from build123d import *

# Parameters (mm, degrees)
SKETCH_1_W          = 100
SKETCH_1_H          = 65
EXTRUDE_1_DEPTH     = 12
SKETCH_2_R          = 3.5
CUT_EXTRUDE_2_DEPTH = 10
SKETCH_3_R          = 3.5
CUT_EXTRUDE_3_DEPTH = 61.466933112
SKETCH_4_R          = 3.5
CUT_EXTRUDE_4_DEPTH = 61.466933112
CUT_EXTRUDE_5_REACH = 84.879
SKETCH_5_R          = 1.5
CUT_EXTRUDE_6_REACH = 84.879
SKETCH_6_R          = 1.5
FILLET_3_R          = 2


with BuildPart() as part:
    # 草图1 → 凸台-拉伸1 (new body)
    with BuildSketch(Plane(origin=(0, 0, 0), x_dir=(1, 0, 0), z_dir=(0, 1, 0))):
        Rectangle(SKETCH_1_W, SKETCH_1_H)
    extrude(amount=EXTRUDE_1_DEPTH)

    # 草图2 → 切除-拉伸2 (cut)
    with BuildSketch(Plane(origin=(0, 12, 0), x_dir=(1, 0, 0), z_dir=(0, 1, 0))):
        with Locations(Location((-40, -9, 0), (0, 0, 270))):
            Circle(SKETCH_2_R)
        with Locations(Location((40, -9, 0), (0, 0, 90))):
            Circle(SKETCH_2_R)
        with BuildLine():
            Line((-30.422291236, 30.788854382), (-33.577708764, 29.211145618))
            ThreePointArc((-33.577708764, 29.211145618), (-34.012630114, 29.053502021), (-34.472135955, 29))
            Line((-34.472135955, 29), (-41, 29))
            ThreePointArc((-41, 29), (-43.828427125, 27.828427125), (-45, 25))
            Line((-45, 25), (-45, 6))
            ThreePointArc((-45, 6), (-43.535533906, 2.464466094), (-40, 1))
            ThreePointArc((-40, 1), (-30, -9), (-40, -19))
            ThreePointArc((-40, -19), (-45, -24), (-40, -29))
            Line((-40, -29), (-34.439229319, -29))
            ThreePointArc((-34.439229319, -29), (-33.976113717, -29.054357705), (-33.538172016, -29.214476061))
            Line((-33.538172016, -29.214476061), (-30.425003094, -30.785523939))
            ThreePointArc((-30.425003094, -30.785523939), (-29.987061393, -30.945642295), (-29.52394579, -31))
            Line((-29.52394579, -31), (29.52394579, -31))
            ThreePointArc((29.52394579, -31), (29.987061393, -30.945642295), (30.425003094, -30.785523939))
            Line((30.425003094, -30.785523939), (33.538172016, -29.214476061))
            ThreePointArc((33.538172016, -29.214476061), (33.976113717, -29.054357705), (34.439229319, -29))
            Line((34.439229319, -29), (40, -29))
            ThreePointArc((40, -29), (45, -24), (40, -19))
            ThreePointArc((40, -19), (30, -9), (40, 1))
            ThreePointArc((40, 1), (43.535533906, 2.464466094), (45, 6))
            Line((45, 6), (45, 25))
            ThreePointArc((45, 25), (43.828427125, 27.828427125), (41, 29))
            Line((41, 29), (34.472135955, 29))
            ThreePointArc((34.472135955, 29), (34.012630114, 29.053502021), (33.577708764, 29.211145618))
            Line((33.577708764, 29.211145618), (30.422291236, 30.788854382))
            ThreePointArc((30.422291236, 30.788854382), (29.987369886, 30.946497979), (29.527864045, 31))
            Line((29.527864045, 31), (-29.527864045, 31))
            ThreePointArc((-29.527864045, 31), (-29.987369886, 30.946497979), (-30.422291236, 30.788854382))
        make_face()
    extrude(amount=-CUT_EXTRUDE_2_DEPTH, mode=Mode.SUBTRACT)

    # 草图3 → 切除-拉伸3 (cut, through all)
    with BuildSketch(Plane(origin=(0, 2, 0), x_dir=(1, 0, 0), z_dir=(0, 1, 0))):
        with Locations(Location((-40, -9, 0), (0, 0, 270))):
            Circle(SKETCH_3_R)
    extrude(amount=-CUT_EXTRUDE_3_DEPTH, mode=Mode.SUBTRACT)

    # 草图4 → 切除-拉伸4 (cut, through all)
    with BuildSketch(Plane(origin=(0, 2, 0), x_dir=(1, 0, 0), z_dir=(0, 1, 0))):
        with Locations(Location((40, -9, 0), (0, 0, 270))):
            Circle(SKETCH_4_R)
    extrude(amount=-CUT_EXTRUDE_4_DEPTH, mode=Mode.SUBTRACT)

    # 草图5 → 切除-拉伸5 (cut, up to next)
    with BuildSketch(Plane.XY.offset(32.5), mode=Mode.PRIVATE) as cut_extrude_5_sk1:
        with Locations((-40, 6)):
            Circle(SKETCH_5_R)
    cut_extrude_5_tool1 = extrude(cut_extrude_5_sk1.sketch, amount=-CUT_EXTRUDE_5_REACH, mode=Mode.PRIVATE) & part.part
    # 草图5 → 切除-拉伸5 (cut, up to next)
    with BuildSketch(Plane.XY.offset(32.5), mode=Mode.PRIVATE) as cut_extrude_5_sk2:
        with Locations((40, 6)):
            Circle(SKETCH_5_R)
    cut_extrude_5_tool2 = extrude(cut_extrude_5_sk2.sketch, amount=-CUT_EXTRUDE_5_REACH, mode=Mode.PRIVATE) & part.part
    add(cut_extrude_5_tool1.solids().sort_by_distance((-40, 6, 32.5))[0], mode=Mode.SUBTRACT)
    add(cut_extrude_5_tool2.solids().sort_by_distance((40, 6, 32.5))[0], mode=Mode.SUBTRACT)

    # 草图6 → 切除-拉伸6 (cut, up to next)
    with BuildSketch(Plane(origin=(0, 0, -32.5), x_dir=(-1, 0, 0), z_dir=(0, 0, -1)), mode=Mode.PRIVATE) as cut_extrude_6_sk1:
        with Locations(Location((-40, 6, 0), (0, 0, 180))):
            Circle(SKETCH_6_R)
    cut_extrude_6_tool1 = extrude(cut_extrude_6_sk1.sketch, amount=-CUT_EXTRUDE_6_REACH, mode=Mode.PRIVATE) & part.part
    # 草图6 → 切除-拉伸6 (cut, up to next)
    with BuildSketch(Plane(origin=(0, 0, -32.5), x_dir=(-1, 0, 0), z_dir=(0, 0, -1)), mode=Mode.PRIVATE) as cut_extrude_6_sk2:
        with Locations(Location((40, 6, 0), (0, 0, 180))):
            Circle(SKETCH_6_R)
    cut_extrude_6_tool2 = extrude(cut_extrude_6_sk2.sketch, amount=-CUT_EXTRUDE_6_REACH, mode=Mode.PRIVATE) & part.part
    add(cut_extrude_6_tool1.solids().sort_by_distance((40, 6, -32.5))[0], mode=Mode.SUBTRACT)
    add(cut_extrude_6_tool2.solids().sort_by_distance((-40, 6, -32.5))[0], mode=Mode.SUBTRACT)

    # 圆角3
    fillet_3_edges = [part.edges().sort_by_distance(p)[0] for p in [
        (-50, 12, 0),
        (50, 12, 0),
    ]]
    fillet(fillet_3_edges, radius=FILLET_3_R)


solid = part.part
Geometry: final body of the model. Coordinates: model frame, mm. A direction names the side the tool comes from. Coordinates: 2 decimals unless noted, no trailing zeros. Order: outer loops, then holes, each group sorted by start corner. A loop starts at its lowest first (then second) coordinate and runs counter-clockwise, first axis right, second up. Notation, with made-up numbers: M -25.75,-8.5 L 33.25,-8.5 A13 ccw 33.25,-4.5 Z; hole C 40.25,12.25 d1. An arc over 180 degrees is marked long. One line per question, with ' | ' between items. Start each with the question number.
Item 1: Draft query along Y for faces 3 (the cylindrical face through (38.5, 6.07, 30.66)), 4 (the flat face through (-32, 12, 7)), 5 (the flat face through (-1, 6, 32.5)), 6 (the cylindrical face through (-41.5, 6.07, 30.66)). Return one class per face: released by +Y, released by -Y, zero draft, split by the parting line, or undercut.
Item 2: Pin query (flat end, axial travel): pin 1 Ø4 at (x, z) = (40, 9) entering from +Y; pin 2 Ø18.5 at (x, z) = (6, -7) entering from +Y; pin 3 Ø1.8 at (x, y) = (-40, 6) entering from -Z. Return the tip coordinate at first contact, or that it passes through.
Item 3: Cut plane B-B, the plane x = 28. Return the cut outline in (y, z), then the cut area to 3 significant figures.
Item 4: Cut plane A-A, the plane z = 9. Return the cut outline in (x, y), then the cut area to 3 significant figures.
Item 5: Cut plane D-D, the plane z = 27. Return the cut outline in (x, y), then the cut area to 3 significant figures.
Item 6: Set-up query: faces 1 (the cylindrical face through (49.4, 11.43, -0.45)), 2 (the flat face through (32, 7, -30)). Return all of +Z, -Z, +X, -X, +Y, -Y with unobstructed straight access to the full face (end or side cutting, diameter ignored); none if empty.
Item 7: Ray query, probe 1 along Y at (x, z) = (40, -29.9); probe 2 along X at (y, z) = (9, -23); probe 3 along Z at (x, y) = (17, 11.75). Return the intervals inside material, ascending. Write a range as [from, to].
Item 8: Cut plane C-C, the plane y = 6. Count the separate pieces of the cut face and the enclosed holes in it, then the cut area to 3 significant figures.
A:
1) face 3: undercut | face 4: released by +Y | face 5: zero draft | face 6: undercut
2) pin 1: passes through | pin 2: stops at y = 2 | pin 3: stops at z = -1.08
3) outline: M 0,-32.5 L 12,-32.5 L 12,-31 L 2,-31 L 2,31 L 12,31 L 12,32.5 L 0,32.5 Z | area: 160 mm2
4) outline: M -50,0 L -43.5,0 L -43.5,12 L -48,12 A2 ccw -50,10 Z; M -36.5,0 L 36.5,0 L 36.5,12 L 30,12 L 30,2 L -30,2 L -30,12 L -36.5,12 Z; M 43.5,0 L 50,0 L 50,10 A2 ccw 48,12 L 43.5,12 Z | area: 430 mm2
5) outline: M -50,0 L 50,0 L 50,10 A2 ccw 48,12 L 44,12 L 44,2 L -44,2 L -44,12 L -48,12 A2 ccw -50,10 Z | area: 318 mm2
6) face 1: +Z, -Z, +X, +Y | face 2: +Y
7) probe 1: y = [0, 4.5], [7.5, 12] | probe 2: x = [-50, -45], [45, 50] | probe 3: z = [-32.5, -31], [31, 32.5]
8) separate pieces: 4 | enclosed holes: 2 | area: 1,460 mm2
